The model under review builds one solid part; all positions refer to its coordinate system, in mm. A direction names the side the tool comes from. Give positions to 0.01 mm unless a question says otherwise; leave off trailing zeros. Order: outer loops, then holes, each group sorted by start corner. A loop starts at its lowest first (then second) coordinate and runs counter-clockwise, first axis right, second up. Notation, with made-up numbers: (89, 87) - (97, 87) arc R14 ccw to (97, 112) - close; hole circle Ø2 at (17, 60.25). An arc over 180 degrees is marked (long way). Use CSV: the item, a comma, the result in double quotes. Start each with the question number.
```python
from build123d import *

# Parameters (mm, degrees)
BOSS_EXTRUDE1_DEPTH = 9.5
FILLET1_R           = 3


with BuildPart() as part:
    # Sketch1 → Boss-Extrude1 (new body, symmetric)
    with BuildSketch(Plane.XY):
        Polygon((-32.5, 2.3), (32.5, 2.3), (32.5, 0.7), (17.5, 0.7), (17.5, -0.7), (19.784478645, 0.584636857), (32.5, 0.584636857), (32.5, -1.015363143), (19.784478645, -1.015363143), (17.5, -2.3), (-32.5, -2.3), align=None)
    extrude(amount=BOSS_EXTRUDE1_DEPTH, both=True)

    # Fillet1
    fillet1_edges = [part.edges().sort_by_distance(p)[0] for p in [
        (32.5, 1.5, -9.5),
        (32.5, -0.215363143, -9.5),
        (32.5, 1.5, 9.5),
        (32.5, -0.215363143, 9.5),
    ]]
    fillet(fillet1_edges, radius=FILLET1_R)


solid = part.part
```
1. Clearance check with a flat-ended pin moving along its axis: pin 1 (7.5 mm diameter, centred on x = 25.5, z = -3, fed in from -Y). State where the tip first meets the part, or that it passes through.
2. Mouldability with a two-part tool opening along Y and no side actions: class faces 1 (the face through (31.6, 1.49, 8.64)), 2 (the face through (18.626, -0.067, 0.133)), 3 (the face through (0, 2.3, 0)) as pulls with the +Y half, pulls with the -Y half, needs draft (parallel to the pull), parting line crosses it, or undercut.
3. Tool access review of faces 4 (the face through (26, -1.015, 0)), 5 (the face through (31.64, -0.23, -8.6)): name each direction out of +Z, -Z, +X, -X, +Y, -Y from which nothing blocks a thin tool from reaching the whole face with its end or side.
4. Consider section A-A (z = -2.25). Give the boundary of the cut face in (x, y), and give its area (3 significant figures).
5. To check wall thickness, follow L1, parallel to X at y = -0.1, z = -4.5; L2, parallel to X at y = -0.05, z = -4; L3, parallel to X at y = 2, z = -8.5. State the ranges of each line that lie inside material, in increasing order. Write a range as [from, to].
Answers follow:
1,pin 1,"stops at y = -1.02"
2,face 1,"needs draft"
2,face 2,"undercut"
2,face 3,"pulls with the +Y half"
3,face 4,"+Z, -Z, +X, -Y"
3,face 5,"-Z, +X, +Y, -Y"
4,outline,"(-32.5, -2.3) - (17.5, -2.3) - (19.78, -1.02) - (32.5, -1.02) - (32.5, 0.58) - (19.78, 0.58) - (17.5, -0.7) - (17.5, 0.7) - (32.5, 0.7) - (32.5, 2.3) - (-32.5, 2.3) - close"
4,area,"278 mm^2"
5,L1,"x = [-32.5, 17.5], [18.57, 32.5]"
5,L2,"x = [-32.5, 17.5], [18.66, 32.5]"
5,L3,"x = [-32.5, 31.74]"
